The figure shows three views and two pictorial views of one solid part (mm, origin at its lowest corner). Answer the questions. A direction names the side the tool comes from. Round coordinates to 2 decimals unless told otherwise and drop trailing zeros. Order: outer loops, then holes, each group sorted by start corner. A loop starts at its lowest first (then second) coordinate and runs counter-clockwise, first axis right, second up. Notation, with made-up numbers: (41, 65) -> (97, 65) arc R33 cw to (97, 93) -> close; hole circle Ø3 at (53, 77.25). An arc over 180 degrees is marked (long way). Answer as a JSON object with one key per item and string values. Group by question number.
Item 1: Section C-C, the plane y = 29 is taken. Write down the section's boundary in (x, z).
Item 2: The mould has two halves that part along X. Classify the marked faces 3, 4, 5 and 6: pulls with the +X half, pulls with the -X half, needs draft (parallel to the pull), parting line crosses it, or undercut.
Item 3: Consider probe 1 along X at (y, z) = (30, 23); probe 2 along X at (y, z) = (22, 38.5); probe 3 along X at (y, z) = (21, 33.5). Determine where each line is inside the solid, lowest interval first. Write a range as from..to.
Item 4: Section A-A, the plane y = 43 is taken. Write down the section's boundary in (x, z), plus the area to 3 significant figures.
Item 5: Section D-D, the plane z = 18.5 is taken. Write down the section's boundary in (x, y).
Item 6: For the marked faces 1 and 2, determine the directions among +Z, -Z, +X, -X, +Y, -Y from which every point of the face is accessible in a straight line to the end or side of a thin tool.
Item 7: Section B-B, the plane z = 33 is taken. Write down the section's boundary in (x, y), plus the area to 3 significant figures.
Item 8: Given P1, Ø6, axis at x = 38.5, y = 29, coming from the -Z side; P2, Ø1.5, axis at y = 41.5, z = 38.5, coming from the -X side; P3, Ø3, axis at x = 12.5, y = 29.5, coming from the -Z side; P4, Ø13, axis at y = 29, z = 7, coming from the +X side, each flat-ended and moving along its own axis, determine where each tip first touches the part or whether it passes through.
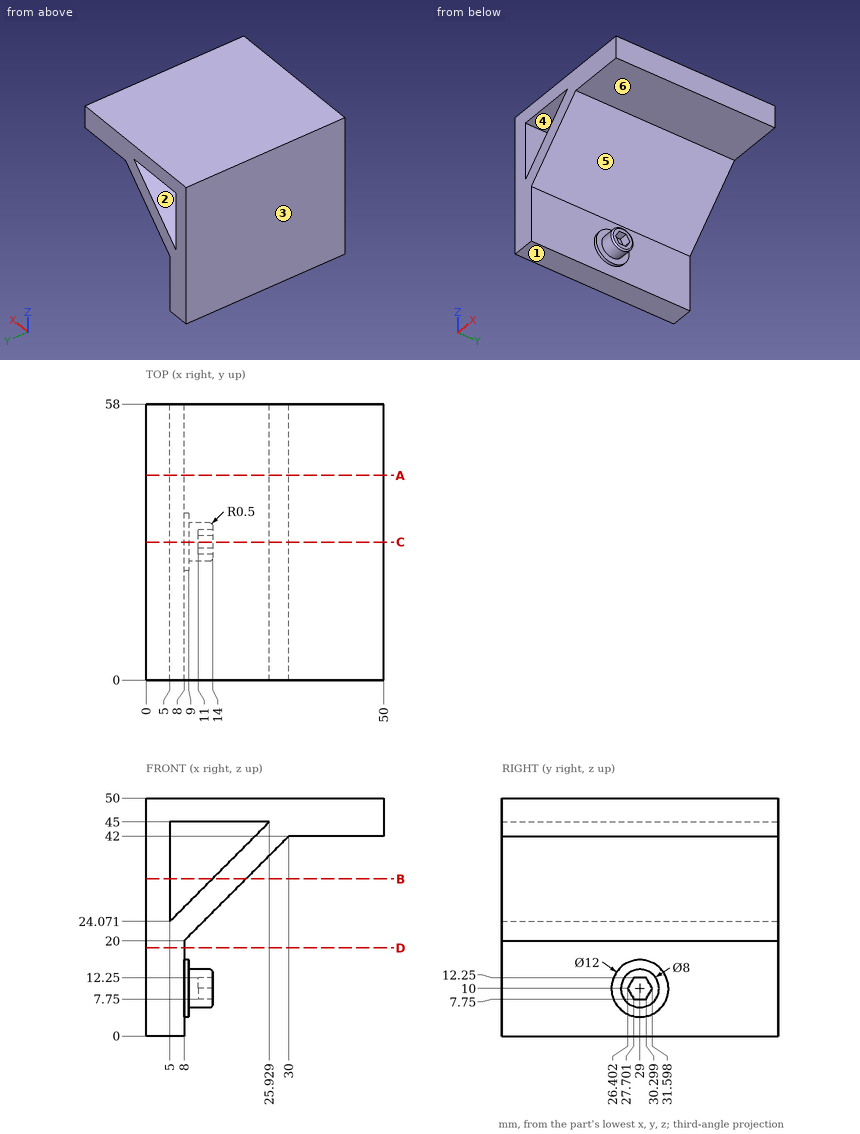
Values found:
{
 "1": {"outline": "(0, 0) -> (8, 0) -> (8, 4) -> (9, 4) -> (9, 6) -> (13.5, 6) arc R0.5 ccw to (14, 6.5) -> (14, 7.75) -> (11, 7.75) -> (11, 12.25) -> (14, 12.25) -> (14, 13.5) arc R0.5 ccw to (13.5, 14) -> (9, 14) -> (9, 16) -> (8, 16) -> (8, 20) -> (30, 42) -> (50, 42) -> (50, 50) -> (0, 50) -> close; hole (5, 24.07) -> (25.93, 45) -> (5, 45) -> close"},
 "2": {"face 3": "pulls with the -X half", "face 4": "undercut", "face 5": "pulls with the +X half", "face 6": "needs draft"},
 "3": {"probe 1": "0..11", "probe 2": "0..5, 19.43..26.5", "probe 3": "0..5, 14.43..21.5"},
 "4": {"outline": "(0, 0) -> (8, 0) -> (8, 20) -> (30, 42) -> (50, 42) -> (50, 50) -> (0, 50) -> close; hole (5, 24.07) -> (25.93, 45) -> (5, 45) -> close", "area": "759 mm2"},
 "5": {"outline": "(0, 0) -> (8, 0) -> (8, 58) -> (0, 58) -> close"},
 "6": {"face 1": "-Z, +X, -X, +Y, -Y", "face 2": "+Y, -Y"},
 "7": {"outline": "(0, 0) -> (5, 0) -> (5, 58) -> (0, 58) -> close; (13.93, 0) -> (21, 0) -> (21, 58) -> (13.93, 58) -> close", "area": "700 mm2"},
 "8": {"P1": "z = 42", "P2": "x = 0", "P3": "z = 6", "P4": "x = 14"}
}
